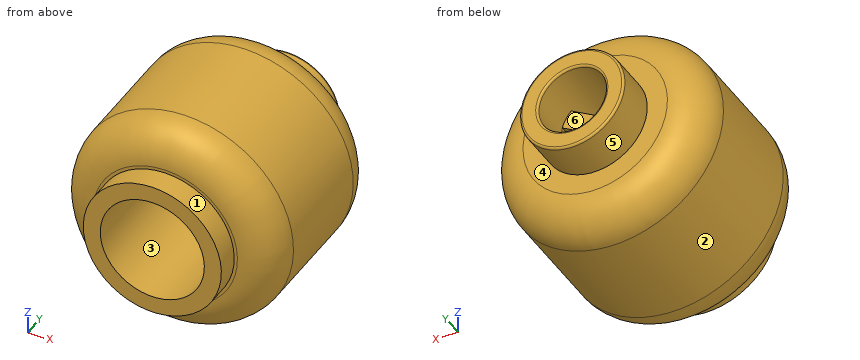
```python
from build123d import *

# Parameters (mm, degrees)
SKETCH2_R           = 5.1
BOSS_EXTRUDE1_DEPTH = 8.5
SKETCH3_R           = 2.45
BOSS_EXTRUDE2_DEPTH = 2
SKETCH4_R           = 1.6
CUT_EXTRUDE1_DEPTH  = 2
FILLET1_R           = 1.7
FILLET2_R           = 0.1
SKETCH5_R           = 3.25
BOSS_EXTRUDE3_DEPTH = 1.1
SKETCH6_R           = 2.45
CUT_EXTRUDE2_DEPTH  = 8.5
CUT_EXTRUDE3_DEPTH  = 1.1


with BuildPart() as part:
    # Sketch2 → Boss-Extrude1 (new body)
    with BuildSketch(Plane(origin=(0, 0, 0), x_dir=(1, 0, 0), z_dir=(0, 1, 0))):
        with Locations(Location((0, 0, 0), (0, 0, 270))):
            Circle(SKETCH2_R)
    extrude(amount=BOSS_EXTRUDE1_DEPTH)

    # Sketch3 → Boss-Extrude2 (add)
    with BuildSketch(Plane(origin=(0, 8.5, 0), x_dir=(1, 0, 0), z_dir=(0, 1, 0))):
        with Locations(Location((0, 0, 0), (0, 0, 270))):
            Circle(SKETCH3_R)
    extrude(amount=BOSS_EXTRUDE2_DEPTH)

    # Sketch4 → Cut-Extrude1 (cut)
    with BuildSketch(Plane(origin=(0, 10.5, 0), x_dir=(1, 0, 0), z_dir=(0, 1, 0))):
        with Locations(Location((0, 0, 0), (0, 0, 270))):
            Circle(SKETCH4_R)
    extrude(amount=-CUT_EXTRUDE1_DEPTH, mode=Mode.SUBTRACT)

    # Fillet1
    fillet1_edges = [part.edges().sort_by_distance(p)[0] for p in [
        (0, 0, -5.1),
        (0, 8.5, -5.1),
    ]]
    fillet(fillet1_edges, radius=FILLET1_R)

    # Fillet2
    fillet2_edges = [part.edges().sort_by_distance(p)[0] for p in [
        (0, 10.5, -1.6),
        (0, 10.5, -2.45),
    ]]
    fillet(fillet2_edges, radius=FILLET2_R)

    # Sketch5 → Boss-Extrude3 (add)
    with BuildSketch(Plane.XZ):
        with Locations(Location((0, 0, 0), (0, 0, 90))):
            Circle(SKETCH5_R)
    extrude(amount=BOSS_EXTRUDE3_DEPTH)

    # Sketch6 → Cut-Extrude2 (cut)
    with BuildSketch(Plane.XZ.offset(1.1)):
        with Locations(Location((0, 0, 0), (0, 0, 90))):
            Circle(SKETCH6_R)
    extrude(amount=-CUT_EXTRUDE2_DEPTH, mode=Mode.SUBTRACT)

    # Sketch11 → Cut-Extrude3 (cut)
    with BuildSketch(Plane(origin=(0, 8.5, 0), x_dir=(1, 0, 0), z_dir=(0, 1, 0))):
        with BuildLine():
            Line((-0.42, 0.240604968), (-0.42, 1.543891188))
            ThreePointArc((-0.42, 1.543891188), (-1.386062698, 0.799268539), (-1.546617211, -0.409847781))
            Line((-1.546617211, -0.409847781), (-0.42, 0.240604968))
        make_face()
        with BuildLine():
            ThreePointArc((1.6, 0), (1.271219887, 0.971596624), (0.42, 1.543891188))
            Line((0.42, 1.543891188), (0.42, 0.240604968))
            Line((0.42, 0.240604968), (1.546617211, -0.409847781))
            ThreePointArc((1.546617211, -0.409847781), (1.586598175, -0.206654861), (1.6, 0))
        make_face()
        with BuildLine():
            Line((0, -0.486856371), (-1.125849182, -1.136865699))
            ThreePointArc((-1.125849182, -1.136865699), (0, -1.6), (1.125849182, -1.136865699))
            Line((1.125849182, -1.136865699), (0, -0.486856371))
        make_face()
    extrude(amount=-CUT_EXTRUDE3_DEPTH, mode=Mode.SUBTRACT)


solid = part.part
```
Verification items for the finished model (mm, model axes). Face numbers are marked on the shaded views. A direction names the side the tool comes from. Coordinates: 2 decimals unless noted, no trailing zeros. Order: outer loops, then holes, each group sorted by start corner. A loop starts at its lowest first (then second) coordinate and runs counter-clockwise, first axis right, second up. Notation, with made-up numbers: (-29, 79) -> (-4, 79) arc R17 cw to (-4, 101) -> close; hole circle Ø10 at (-8, -22). An arc over 180 degrees is marked (long way). Put each result on its own line as item: value. Start each with the question number.
1) Material ranges on L1, parallel to X at y = 9.3, z = 0; L2, parallel to X at y = 8.3, z = 0; L3, parallel to X at y = 8.1, z = 0, recorded low to high.
2) Go/stop test with flat-tipped pins: pin 1 (1.5 mm diameter, centred on x = -3, y = 4, fed in from +Z); pin 2 (5 mm diameter, centred on x = 4, z = 3.5, fed in from +Y); pin 3 (1.5 mm diameter, centred on x = -3, z = -4, fed in from +Y). Record where each tip stops, or that it passes through.
3) Cross-section at B-B (z = 0.25). State how many separate pieces and enclosed holes the cut face has, plus the area to 3 significant figures.
4) Cross-section at A-A (y = 6.5). Enter the section's corners in (x, z).
5) Tool access check on the marked faces 1 and 2. Record the directions out of +Z, -Z, +X, -X, +Y, -Y that give a thin tool (end or side, any length) a straight path to the whole face; none if there is none.
6) Release check for a two-part mould opening along Z. For the marked faces 3, 4, 5 and 6 record: pulls with the +Z half, pulls with the -Z half, needs draft (parallel to the pull), parting line crosses it, or undercut.
Geometry check:
1. L1: x = -2.45 to -1.6, 1.6 to 2.45
1. L2: x = -4.2 to -1.6, -0.84 to 0.84, 1.6 to 4.2
1. L3: x = -4.5 to -1.6, -0.84 to 0.84, 1.6 to 4.5
2. pin 1: stops at z = 4.58
2. pin 2: stops at y = 8.5
2. pin 3: stops at y = 8.27
3. separate pieces: 3
3. enclosed holes: 0
3. area: 52.5 mm^2
4. outline: circle Ø10.2 at (0, 0); hole circle Ø4.9 at (0, 0)
5. face 1: -Y
5. face 2: +Y, -Y
6. face 3: undercut
6. face 4: needs draft
6. face 5: parting line crosses it
6. face 6: undercut
